The model under review builds one solid part; all positions refer to its coordinate system, in mm. A direction names the side the tool comes from. Give positions to 0.01 mm unless a question says otherwise; leave off trailing zeros. Loops run counter-clockwise (first coordinate to the right, second up) from the corner with the lowest first, then second, coordinate; pieces in that order, holes last. Notation, with made-up numbers: M 7,-25.75 L 19,-25.75 A21 cw 19,5.25 Z; hole C 17.25,-19 d7. An arc over 180 degrees is marked long. Return JSON: item names as keys, results as strings.
```python
from build123d import *
from OCP.BRepFilletAPI import BRepFilletAPI_MakeChamfer

# Parameters (mm, degrees)
SKETCH1_W           = 203.2
SKETCH1_H           = 63.5
SKETCH1_R           = 1.27
BOSS_EXTRUDE1_DEPTH = 2.54
SKETCH2_W           = 86.36
SKETCH2_H           = 20.32
SKETCH2_R           = 2.54
BOSS_EXTRUDE2_DEPTH = 2.54
SKETCH3_W           = 3.81
SKETCH3_H           = 25.4
BOSS_EXTRUDE3_DEPTH = 17.78
CHAMFER1_SIZE       = 17.62
CHAMFER1_SIZE2      = 23.382529757
SKETCH4_W           = 35.56
SKETCH4_H           = 35.56
CUT_EXTRUDE1_DEPTH  = 214.631969518
FILLET1_R           = 10
BOSS_EXTRUDE4_DEPTH = 17.78
FILLET2_R           = 12.54


with BuildPart() as part:
    # Sketch1 → Boss-Extrude1 (new body)
    with BuildSketch(Plane(origin=(0, 0, 0), x_dir=(1, 0, 0), z_dir=(0, 1, 0))):
        with Locations((101.6, 31.75)):
            Rectangle(SKETCH1_W, SKETCH1_H)
        with Locations(Location((7.62, 55.88, 0), (0, 0, 270))):
            Circle(SKETCH1_R, mode=Mode.SUBTRACT)
        with Locations(Location((55.88, 55.88, 0), (0, 0, 270))):
            Circle(SKETCH1_R, mode=Mode.SUBTRACT)
        with Locations(Location((7.62, 7.62, 0), (0, 0, 270))):
            Circle(SKETCH1_R, mode=Mode.SUBTRACT)
        with Locations(Location((55.88, 7.62, 0), (0, 0, 270))):
            Circle(SKETCH1_R, mode=Mode.SUBTRACT)
        with Locations(Location((77.47, 55.88, 0), (0, 0, 270))):
            Circle(SKETCH1_R, mode=Mode.SUBTRACT)
        with Locations(Location((125.73, 55.88, 0), (0, 0, 270))):
            Circle(SKETCH1_R, mode=Mode.SUBTRACT)
        with Locations(Location((125.73, 7.62, 0), (0, 0, 270))):
            Circle(SKETCH1_R, mode=Mode.SUBTRACT)
        with Locations(Location((77.47, 7.62, 0), (0, 0, 270))):
            Circle(SKETCH1_R, mode=Mode.SUBTRACT)
        with Locations(Location((147.32, 55.88, 0), (0, 0, 270))):
            Circle(SKETCH1_R, mode=Mode.SUBTRACT)
        with Locations(Location((195.58, 55.88, 0), (0, 0, 270))):
            Circle(SKETCH1_R, mode=Mode.SUBTRACT)
        with Locations(Location((195.58, 7.62, 0), (0, 0, 270))):
            Circle(SKETCH1_R, mode=Mode.SUBTRACT)
        with Locations(Location((147.32, 7.62, 0), (0, 0, 270))):
            Circle(SKETCH1_R, mode=Mode.SUBTRACT)
    extrude(amount=BOSS_EXTRUDE1_DEPTH)

    # Sketch2 → Boss-Extrude2 (add)
    with BuildSketch(Plane.XY):
        with Locations((101.6, -7.62)):
            Rectangle(SKETCH2_W, SKETCH2_H)
        with Locations((66.675, -7.62)):
            Circle(SKETCH2_R, mode=Mode.SUBTRACT)
        with Locations((136.525, -7.62)):
            Circle(SKETCH2_R, mode=Mode.SUBTRACT)
    extrude(amount=-BOSS_EXTRUDE2_DEPTH)

    # Sketch3 → Boss-Extrude3 (add)
    with BuildSketch(Plane.XZ):
        with Locations((60.325, -15.24)):
            Rectangle(SKETCH3_W, SKETCH3_H)
        with Locations((142.875, -15.24)):
            Rectangle(SKETCH3_W, SKETCH3_H)
    extrude(amount=BOSS_EXTRUDE3_DEPTH)

    # Chamfer1: one chamfer whose edges measure the first distance from different faces: ONE call of the kernel's chamfer builder (chamfer() names one face for all edges)
    chamfer1_edges_1 = [part.edges().sort_by_distance(p)[0] for p in [
        (142.875, -17.78, -27.94),
    ]]
    chamfer1_side_1 = [part.faces().sort_by_distance(p)[0] for p in [
        (142.875, -8.89, -27.94),
    ]]
    chamfer1_edges_2 = [part.edges().sort_by_distance(p)[0] for p in [
        (60.325, -17.78, -27.94),
    ]]
    chamfer1_side_2 = [part.faces().sort_by_distance(p)[0] for p in [
        (60.325, -8.89, -27.94),
    ]]
    chamfer1 = BRepFilletAPI_MakeChamfer(part.part.solid().wrapped)
    for e in chamfer1_edges_1:
        chamfer1.Add(CHAMFER1_SIZE, CHAMFER1_SIZE2, e.wrapped, chamfer1_side_1[0].wrapped)  # the first distance lies on this face
    for e in chamfer1_edges_2:
        chamfer1.Add(CHAMFER1_SIZE, CHAMFER1_SIZE2, e.wrapped, chamfer1_side_2[0].wrapped)  # the first distance lies on this face
    add(Compound.cast(chamfer1.Shape()), mode=Mode.REPLACE)

    # Sketch4 → Cut-Extrude1 (cut, through all)
    with BuildSketch(Plane.XZ):
        with Locations((31.75, -31.75)):
            Rectangle(SKETCH4_W, SKETCH4_H)
        with Locations((101.6, -31.75)):
            Rectangle(SKETCH4_W, SKETCH4_H)
        with Locations((171.45, -31.75)):
            Rectangle(SKETCH4_W, SKETCH4_H)
    extrude(amount=-CUT_EXTRUDE1_DEPTH, mode=Mode.SUBTRACT)

    # Fillet1
    fillet1_edges = [part.edges().sort_by_distance(p)[0] for p in [
        (13.97, 1.27, -49.53),
        (13.97, 1.27, -13.97),
        (49.53, 1.27, -13.97),
        (49.53, 1.27, -49.53),
        (83.82, 1.27, -49.53),
        (83.82, 1.27, -13.97),
        (119.38, 1.27, -13.97),
        (119.38, 1.27, -49.53),
        (153.67, 1.27, -49.53),
        (153.67, 1.27, -13.97),
        (189.23, 1.27, -13.97),
        (189.23, 1.27, -49.53),
    ]]
    fillet(fillet1_edges, radius=FILLET1_R)

    # Sketch5 → Boss-Extrude4 (add)
    with BuildSketch(Plane.XZ):
        Polygon((0, 0), (5.08, 0), (11.43, 0), (11.43, -3.81), (5.08, -3.81), (5.08, -15.24), (0, -15.24), align=None)
        Polygon((203.2, 0), (191.77, 0), (191.77, -3.81), (198.12, -3.81), (198.12, -15.24), (203.2, -15.24), align=None)
    extrude(amount=BOSS_EXTRUDE4_DEPTH)

    # Fillet2
    fillet2_edges = [part.edges().sort_by_distance(p)[0] for p in [
        (200.66, -17.78, -15.24),
        (2.54, -17.78, -15.24),
    ]]
    fillet(fillet2_edges, radius=FILLET2_R)


solid = part.part
```
1) Consider section B-B on x = 22. Write out the cut boundary in (y, z).
From the geometry:
{"outline": "M 0,-63.5 L 2.54,-63.5 L 2.54,-49.33 L 0,-49.33 Z; M 0,-14.17 L 2.54,-14.17 L 2.54,0 L 0,0 Z"}
2) Consider section D-D on y = -3.25. Write out the cut boundary in (x, z), then the cut area to 3 significant figures.
From the geometry:
{"outline": "M 0,-15.24 L 5.08,-15.24 L 5.08,-3.81 L 11.43,-3.81 L 11.43,0 L 0,0 Z; M 58.42,-23.84 L 62.23,-23.84 L 62.23,-2.54 L 140.97,-2.54 L 140.97,-23.84 L 144.78,-23.84 L 144.78,0 L 58.42,0 Z; M 191.77,-3.81 L 198.12,-3.81 L 198.12,-15.24 L 203.2,-15.24 L 203.2,0 L 191.77,0 Z", "area": "585 mm²"}
3) Tool access review of faces 3 (the face through (86.67, 1.29, -16.98)), 4 (the face through (191.77, -9, -2)), 5 (the face through (3, -3, -15.24)), 6 (the face through (101, -9, -2.54)): name each direction out of +Z, -Z, +X, -X, +Y, -Y from which nothing blocks a thin tool from reaching the whole face with its end or side.
From the geometry:
{"face 3": "+Y, -Y", "face 4": "+Z, -Z, -Y", "face 5": "-Z, -X, -Y", "face 6": "-Z, -Y"}
4) The part is to be moulded in two halves that separate along X. For faces 1 (the face through (116.37, 1.29, -16.82)), 2 (the face through (126, -7, 0)), say which applies: released by +X, released by -X, zero draft, split by the parting line, or undercut.
From the geometry:
{"face 1": "undercut", "face 2": "zero draft"}
5) Insertion check: pin 1 (3 mm diameter, centred on x = 63.5, z = -10.5, fed in from -Y); pin 2 (1.5 mm diameter, centred on x = 143.5, y = -7.5, fed in from -Z); pin 3 (5.5 mm diameter, centred on x = 3.5, y = -3, fed in from -Z). Each pin has a flat end and moves straight along its axis. Give the tip position at first contact, or say it passes through.
From the geometry:
{"pin 1": "y = -13.9", "pin 2": "z = -19.19", "pin 3": "z = -15.24"}
6) Wall thickness on L1, parallel to X at y = -9.25, z = -7; L2, parallel to Z at x = 195.58, y = 1.5; L3, parallel to Z at x = 57, y = 1.25: over which ranges is each line inside the solid? List them lowest first. Write a range as from..to.
From the geometry:
{"L1": "0..5.08, 58.42..62.23, 140.97..144.78, 198.12..203.2", "L2": "-63.5..-57.15, -54.61..-8.89, -6.35..0", "L3": "-63.5..-56.48, -55.28..-8.22, -7.02..0"}
7) Consider section A-A on y = -14.5. Write out the cut boundary in (x, z).
From the geometry:
{"outline": "M 0,-11.16 L 5.08,-11.16 L 5.08,-3.81 L 11.43,-3.81 L 11.43,0 L 0,0 Z; M 58.42,-8.91 L 62.23,-8.91 L 62.23,-2.54 L 140.97,-2.54 L 140.97,-8.91 L 144.78,-8.91 L 144.78,0 L 58.42,0 Z; M 191.77,-3.81 L 198.12,-3.81 L 198.12,-11.16 L 203.2,-11.16 L 203.2,0 L 191.77,0 Z"}
8) Consider section C-C on z = -18.5. Write out the cut boundary in (x, y), then the cut area to 3 significant figures.
From the geometry:
{"outline": "M 0,0 L 15.6,0 L 15.6,2.54 L 0,2.54 Z; M 47.9,0 L 58.42,0 L 58.42,-7.27 L 62.23,-7.27 L 62.23,0 L 85.45,0 L 85.45,2.54 L 47.9,2.54 Z; M 117.75,0 L 140.97,0 L 140.97,-7.27 L 144.78,-7.27 L 144.78,0 L 155.3,0 L 155.3,2.54 L 117.75,2.54 Z; M 187.6,0 L 203.2,0 L 203.2,2.54 L 187.6,2.54 Z", "area": "325 mm²"}
